Check sheet for the modelled part. Datum: model origin and axes. Units: mm. Face numbers are marked on the shaded views. A direction names the side the tool comes from. Round coordinates to 2 decimals unless told otherwise and drop trailing zeros. Loops run counter-clockwise (first coordinate to the right, second up) from the corner with the lowest first, then second, coordinate; pieces in that order, holes last. Notation, with made-up numbers: (-23, 10.25) -> (6, 10.25) arc R26 ccw to (6, 48.25) -> close; hole circle Ø9 at (80, 71.25). An arc over 180 degrees is marked (long way). One line per item, written item: value. Start each with the question number.
1. Cross-section at D-D on y = 59.5. Record the cut outline in (x, z).
2. Cross-section at A-A on y = 7.5. Record the cut outline in (x, z).
3. Cross-section at B-B on x = -507.5. Record the cut outline in (y, z), then the cut area to 3 significant figures.
4. Release check for a two-part mould opening along X. For the marked faces 1, 2 and 3 record: +X half, -X half, draft (parallel to the pull), parting line (faces both ways), or undercut.
5. Material ranges on L1, parallel to X at y = 7.5, z = 5.25; L2, parallel to Y at x = -507.5, z = 6; L3, parallel to Z at x = -470, y = 94, recorded low to high.
6. Set-up check for the marked faces 4, 5, 6, 7 and 8: record each of +Z, -Z, +X, -X, +Y, -Y from which the full face is reachable in a straight line by a thin tool's end or side.
7. Go/stop test with flat-tipped pins: pin 1 (5 mm diameter, centred on y = 21, z = 3.5, fed in from -X); pin 2 (2.5 mm diameter, centred on x = -442.26, y = 7.5, fed in from -Z); pin 3 (5 mm diameter, centred on x = -403.5, z = 6.5, fed in from +Y); pin 4 (3 mm diameter, centred on x = -435, z = 4, fed in from +Y). Record where each tip stops, or that it passes through.
8. Cross-section at C-C on z = 8. Record the cut outline in (x, y).
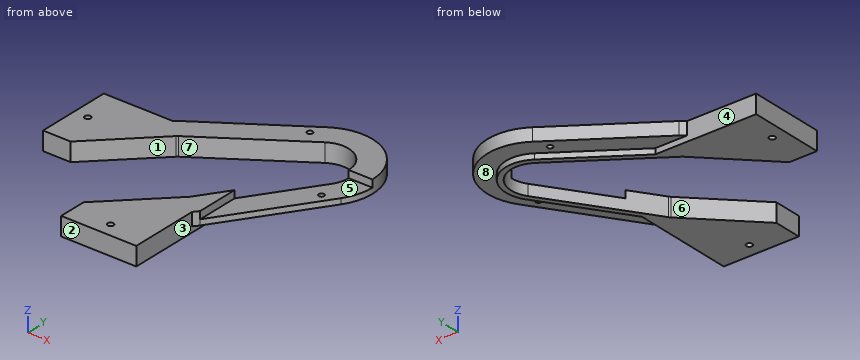
Autodesk Inventor part; units mm, degrees
ref_plane "YZ Plane" through (0, 0, 0) normal (1, 0, 0) x (0, 1, 0)
ref_plane "XZ Plane" through (0, 0, 0) normal (0, 1, 0) x (-1, 0, 0)
ref_plane "XY Plane" through (0, 0, 0) normal (0, 0, 1) x (1, 0, 0)
sketch "Sketch13" plane through (0, 0, 0) normal (0, 0, 1) x (1, 0, 0)
  line L0 (-500, 9) -> (0, 9) construction
  line L1 (0, 9) -> (0, 15)
  line L2 (0, 15) -> (-500, 15)
  line L3 (-500, 9) -> (-500, 15)
  line L4 (6, 15) -> (6, 375)
  line L5 (0, 375) -> (6, 375)
  line L6 (0, 15) -> (0, 375)
  line L7 (0, 15) -> (6, 15)
  line L8 (-506, 375) -> (-506, 15) construction
  line L9 (-506, 15) -> (-500, 15)
  line L10 (-500, 15) -> (-500, 375)
  line L11 (-506, 375) -> (-500, 375)
  line L12 (-463.8988, 17.0711) -> (-473.7868, 17.0711)
  line L13 (-473.7868, 17.0711) -> (-497.9289, 41.2132)
  line L14 (-497.9289, 41.2132) -> (-497.9289, 51.1012)
  line L15 (-497.9289, 51.1012) -> (-466.8985, 82.1316)
  arc A0 (-466.4587, 82.4947) -> (-466.8985, 82.1316) centre (-464.7772, 80.0103) ccw
  line L16 (-466.4587, 82.4947) -> (-415.1076, 117.2506)
  arc A1 (-397.7494, 99.8924) -> (-415.1076, 117.2506) centre (-408.1012, 106.8988) ccw
  line L17 (-397.7494, 99.8924) -> (-432.5053, 48.5413)
  arc A2 (-432.8684, 48.1015) -> (-432.5053, 48.5413) centre (-434.9897, 50.2228) ccw
  line L18 (-432.8684, 48.1015) -> (-463.8988, 17.0711)
  circle A3 centre (-460.0736, 33.7132) radius 4
  circle A4 centre (-438.8604, 54.9264) radius 4
  circle A5 centre (-460.0736, 76.1396) radius 4
  circle A6 centre (-481.2868, 54.9264) radius 4
  circle A7 centre (-460.0736, 54.9264) radius 13
  line L19 (-430.7901, 47.3804) -> (-396.0343, 98.7315)
  arc A8 (-396.0343, 98.7315) -> (-416.2685, 118.9657) centre (-408.1012, 106.8988) ccw
  line L20 (-416.2685, 118.9657) -> (-467.6196, 84.2099)
  arc A9 (-467.6196, 84.2099) -> (-468.363, 83.5961) centre (-464.7772, 80.0103) ccw
  line L21 (-468.363, 83.5961) -> (-500, 51.9591)
  line L22 (-500, 51.9591) -> (-500, 40.3553)
  line L23 (-500, 40.3553) -> (-474.6447, 15)
  line L24 (-474.6447, 15) -> (-463.0409, 15)
  line L25 (-463.0409, 15) -> (-431.4039, 46.637)
  arc A10 (-431.4039, 46.637) -> (-430.7901, 47.3804) centre (-434.9897, 50.2228) ccw
  line L26 (-385.3272, 91.4847) -> (-420.0831, 40.1336)
  arc A11 (-422.2618, 37.4949) -> (-420.0831, 40.1336) centre (-434.9897, 50.2228) ccw
  line L27 (-422.2618, 37.4949) -> (-457.6856, 2.0711)
  line L28 (-457.6856, 2.0711) -> (-480, 2.0711)
  line L29 (-480, 2.0711) -> (-512.9289, 35)
  line L30 (-512.9289, 35) -> (-512.9289, 57.3144)
  line L31 (-512.9289, 57.3144) -> (-477.5051, 92.7382)
  arc A12 (-474.8664, 94.9169) -> (-477.5051, 92.7382) centre (-464.7772, 80.0103) ccw
  line L32 (-474.8664, 94.9169) -> (-423.5153, 129.6728)
  arc A13 (-385.3272, 91.4847) -> (-423.5153, 129.6728) centre (-408.1012, 106.8988) ccw
  line L33 (-422.2618, 37.4949) -> (-422.2618, 0)
  line L34 (-477.5051, 92.7382) -> (-515, 92.7382)
  line L35 (0, 6) -> (-500, 6) construction
  line L36 (-500, 0) -> (-500, 6)
  line L37 (0, 0) -> (-500, 0)
  line L38 (0, 0) -> (0, 6)
  line L39 (-509, 15) -> (-509, 375) construction
  line L40 (-515, 375) -> (-509, 375)
  line L41 (-515, 15) -> (-515, 375)
  line L42 (-515, 15) -> (-509, 15)
  line L43 (-500, 51.9591) -> (-515, 51.9591)
  line L44 (-463.0409, 15) -> (-463.0409, 0)
  point P0 (-422.2618, 15)
  point P1 (-500, 92.7382)
  dimension "d27" = 15
extrude "Extrusion14" add sketch "Sketch13" along normal blind 10 contours L25 A10 L19 A8 L20 A9 L21 L10 L31 A12 L32 A13 L26 A11 L27 L2 | L2 L27 L28 L44 | L27 L33 L2 | L2 L33 L37 L44 L28 L27 | L43 L30 L31 L10 | L31 L30 L43 L41 L34 L10 | L10 L34 L31
sketch "Sketch14" plane through (0, 0, 0) normal (0, 0, -1) x (-1, 0, 0)
  line L0 (467.6196, 84.2099) -> (416.2685, 118.9657)
  arc A0 (468.363, 83.5961) -> (467.6196, 84.2099) centre (464.7772, 80.0103) ccw
  line L1 (500, 51.9591) -> (468.363, 83.5961)
  line L2 (515, 51.9591) -> (500, 51.9591)
  line L3 (515, 92.7382) -> (515, 51.9591)
  line L4 (477.5051, 92.7382) -> (515, 92.7382)
  arc A1 (477.5051, 92.7382) -> (474.8664, 94.9169) centre (464.7772, 80.0103) ccw
  line L5 (423.5153, 129.6728) -> (474.8664, 94.9169)
  arc A2 (423.5153, 129.6728) -> (385.3272, 91.4847) centre (408.1012, 106.8988) ccw
  line L6 (420.0831, 40.1336) -> (385.3272, 91.4847)
  arc A3 (420.0831, 40.1336) -> (422.2618, 37.4949) centre (434.9897, 50.2228) ccw
  line L7 (422.2618, 0) -> (422.2618, 37.4949)
  line L8 (463.0409, 0) -> (422.2618, 0)
  line L9 (463.0409, 15) -> (463.0409, 0)
  line L10 (431.4039, 46.637) -> (463.0409, 15)
  arc A4 (430.7901, 47.3804) -> (431.4039, 46.637) centre (434.9897, 50.2228) ccw
  line L11 (396.0343, 98.7315) -> (430.7901, 47.3804)
  arc A5 (416.2685, 118.9657) -> (396.0343, 98.7315) centre (408.1012, 106.8988) ccw
  arc A6 (421.8736, 127.2472) -> (387.7528, 93.1264) centre (408.1012, 106.8988) ccw
  line L12 (421.8736, 127.2472) -> (473.2247, 92.4914)
  arc A7 (476.2278, 89.8093) -> (473.2247, 92.4914) centre (464.7772, 80.0103) ccw
  line L13 (476.2278, 89.8093) -> (512.0711, 89.8093)
  line L14 (512.0711, 89.8093) -> (512.0711, 54.888)
  line L15 (512.0711, 54.888) -> (501.2132, 54.888)
  line L16 (501.2132, 54.888) -> (470.434, 85.6672)
  arc A8 (470.434, 85.6672) -> (469.2613, 86.6355) centre (464.7772, 80.0103) ccw
  line L17 (469.2613, 86.6355) -> (417.9102, 121.3913)
  arc A9 (417.9102, 121.3913) -> (393.6087, 97.0898) centre (408.1012, 106.8988) ccw
  line L18 (393.6087, 97.0898) -> (428.3645, 45.7387)
  arc A10 (428.3645, 45.7387) -> (429.3328, 44.566) centre (434.9897, 50.2228) ccw
  line L19 (429.3328, 44.566) -> (460.112, 13.7868)
  line L20 (460.112, 13.7868) -> (460.112, 2.9289)
  line L21 (460.112, 2.9289) -> (425.1907, 2.9289)
  line L22 (425.1907, 2.9289) -> (425.1907, 38.7722)
  arc A11 (422.5086, 41.7753) -> (425.1907, 38.7722) centre (434.9897, 50.2228) ccw
  line L23 (422.5086, 41.7753) -> (387.7528, 93.1264)
  line L24 (422.2618, 0) -> (422.2618, 37.4949)
  line L25 (422.2618, 37.4949) -> (422.2618, 54.7554)
  line L26 (477.5051, 92.7382) -> (515, 92.7382)
  line L27 (477.5051, 92.7382) -> (455.0191, 92.7382)
  line L28 (467.6196, 84.2099) -> (416.2685, 118.9657)
  point P0 (0, 0)
  point P1 (460.2446, 92.7382)
  dimension "d32" = 10
extrude "Extrusion15" cut sketch "Sketch14" against normal blind 3 contours L17 A9 L18 L25 L23 A6 L12 L27 | L12 A6 L23 L25 A3 L6 A2 L5 A1 L27
sketch "Sketch15" plane through (0, 0, 10) normal (0, 0, 1) x (1, 0, 0)
  line L0 (-467.6196, 84.2099) -> (-416.2685, 118.9657)
  arc A0 (-396.0343, 98.7315) -> (-416.2685, 118.9657) centre (-408.1012, 106.8988) ccw
  line L1 (-396.0343, 98.7315) -> (-430.7901, 47.3804)
  arc A1 (-431.4039, 46.637) -> (-430.7901, 47.3804) centre (-434.9897, 50.2228) ccw
  line L2 (-431.4039, 46.637) -> (-463.0409, 15)
  line L3 (-463.0409, 15) -> (-463.0409, 0)
  line L4 (-463.0409, 0) -> (-422.2618, 0)
  line L5 (-422.2618, 0) -> (-422.2618, 37.4949)
  arc A2 (-422.2618, 37.4949) -> (-420.0831, 40.1336) centre (-434.9897, 50.2228) ccw
  line L6 (-420.0831, 40.1336) -> (-385.3272, 91.4847)
  arc A3 (-385.3272, 91.4847) -> (-423.5153, 129.6728) centre (-408.1012, 106.8988) ccw
  line L7 (-423.5153, 129.6728) -> (-474.8664, 94.9169)
  arc A4 (-474.8664, 94.9169) -> (-477.5051, 92.7382) centre (-464.7772, 80.0103) ccw
  line L8 (-477.5051, 92.7382) -> (-515, 92.7382)
  line L9 (-515, 92.7382) -> (-515, 51.9591)
  line L10 (-515, 51.9591) -> (-500, 51.9591)
  line L11 (-500, 51.9591) -> (-468.363, 83.5961)
  arc A5 (-467.6196, 84.2099) -> (-468.363, 83.5961) centre (-464.7772, 80.0103) ccw
  line L12 (-396.0343, 98.7315) -> (-430.7901, 47.3804)
  line L13 (-420.0831, 40.1336) -> (-385.3272, 91.4847)
  line L14 (-420.0831, 63.1999) -> (-420.0831, 40.1336)
  arc A6 (-396.0343, 98.7315) -> (-416.2685, 118.9657) centre (-408.1012, 106.8988) ccw
  line L15 (-393.5302, 106.8988) -> (-380.6012, 106.8988)
  arc A7 (-385.3272, 91.4847) -> (-423.5153, 129.6728) centre (-408.1012, 106.8988) ccw
  point P0 (0, 0)
extrude "Extrusion16" cut sketch "Sketch15" against normal blind 4 contours L15 A3 L6 L14 L1 A0
sketch "Sketch16" plane through (0, 0, 3) normal (0, 0, -1) x (-1, 0, 0)
  line L0 (420.0831, 40.1336) -> (385.3272, 91.4847)
  arc A0 (423.5153, 129.6728) -> (385.3272, 91.4847) centre (408.1012, 106.8988) ccw
  line L1 (423.5153, 129.6728) -> (474.8664, 94.9169)
  point P0 (0, 0)
  point P1 (393.3272, 88.4847)
  point P2 (426.5153, 121.6728)
  dimension "d37" = 8
  dimension "d38" = 3
  dimension "d39" = 8
  dimension "d40" = 3
hole "Hole1" at (-393.3272, 88.4847, 3) at (-426.5153, 121.6728, 3) direction (0, 0, 1) diameter 2.9 end through all
sketch "Sketch17" plane through (0, 0, 10) normal (0, 0, 1) x (1, 0, 0)
  line L0 (-422.2618, 0) -> (-422.2618, 37.4949)
  line L1 (-477.5051, 92.7382) -> (-515, 92.7382)
  point P0 (0, 0)
  point P1 (-442.2618, 7.5)
  point P2 (-507.5, 72.7382)
  point P3 (-422.2618, 18.7474)
  dimension "d48" = 7.5
  dimension "d49" = 7.5
  dimension "d50" = 20
  dimension "d51" = 20
hole "Hole2" at (-442.2618, 7.5, 10) at (-507.5, 72.7382, 10) direction (0, 0, -1) diameter 3.2 end through all
properties part number "Front Right Cover Bracket" material "ABS Plastic"
Taken from the geometry:
1. outline: (-515, 0) -> (-492.46, 0) -> (-492.46, 10) -> (-515, 10) -> close; (-422.59, 0) -> (-419.05, 0) -> (-419.05, 3) -> (-406.98, 3) -> (-406.98, 6) -> (-420.08, 6) -> (-420.08, 10) -> (-422.59, 10) -> close
2. outline: (-463.04, 0) -> (-443.86, 0) -> (-443.86, 10) -> (-463.04, 10) -> close; (-440.66, 0) -> (-422.26, 0) -> (-422.26, 10) -> (-440.66, 10) -> close
3. outline: (51.96, 0) -> (71.14, 0) -> (71.14, 10) -> (51.96, 10) -> close; (74.34, 0) -> (92.74, 0) -> (92.74, 10) -> (74.34, 10) -> close
3. area: 376 mm2
4. face 1: undercut
4. face 2: draft
4. face 3: +X half
5. L1: x = -463.04 to -443.86, -440.66 to -422.26
5. L2: y = 51.96 to 71.14, 74.34 to 92.74
5. L3: z = 3 to 10
6. face 4: -Z, -X, +Y
6. face 5: +Z, +X, -Y
6. face 6: +Z, -Z, -X
6. face 7: +Z, -Z
6. face 8: -Z
7. pin 1: stops at x = -459.54
7. pin 2: passes through
7. pin 3: stops at y = 134.32
7. pin 4: stops at y = 122.91
8. outline: (-515, 51.96) -> (-500, 51.96) -> (-468.36, 83.6) arc R5.07 cw to (-467.62, 84.21) -> (-416.27, 118.97) arc R14.57 cw to (-393.53, 106.9) -> (-380.6, 106.9) arc R27.5 ccw to (-423.52, 129.67) -> (-474.87, 94.92) arc R18 ccw to (-477.51, 92.74) -> (-515, 92.74) -> close; (-463.04, 0) -> (-422.26, 0) -> (-422.26, 37.49) arc R18 ccw to (-420.08, 40.13) -> (-420.08, 63.2) -> (-430.79, 47.38) arc R5.07 cw to (-431.4, 46.64) -> (-463.04, 15) -> close; hole circle Ø3.2 at (-507.5, 72.74); hole circle Ø3.2 at (-442.26, 7.5); hole circle Ø2.9 at (-426.52, 121.67)
